Check sheet for the drawn part. Datum: minimum x, y, z corner. Units: mm. A direction names the side the tool comes from. Round coordinates to 2 decimals unless told otherwise and drop trailing zeros. Write each loop counter-clockwise with the first axis right and the second up, starting at its lowest first coordinate (ties: lowest second). Pieces come first, ordered by that corner, then holes. Notation, with made-up numbers: (56.25, 8) -> (65.25, 8) arc R15 cw to (65.25, 29) -> close; hole circle Ø5 at (79, -36). An arc over 180 degrees is marked (long way). Use a Markdown table: item, result.
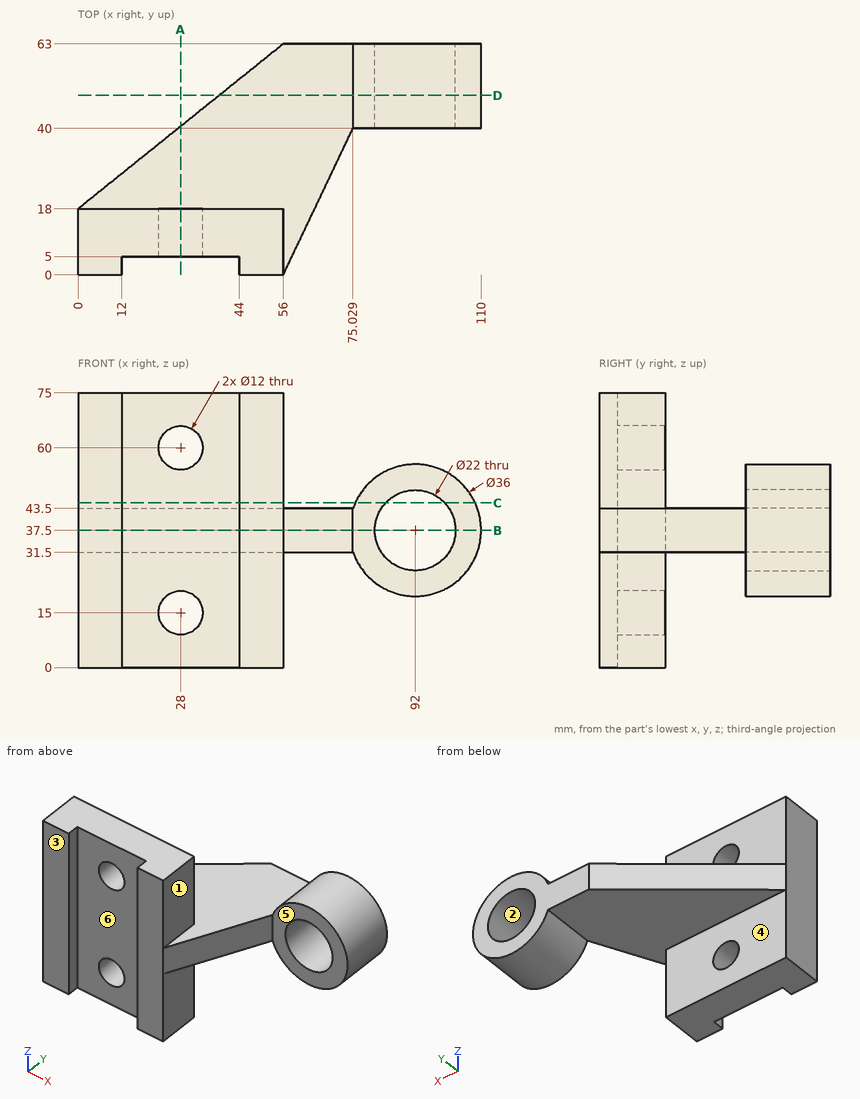
(1) Release check for a two-part mould opening along X. For the marked faces 1, 2 and 3 record: +X half, -X half, draft (parallel to the pull), parting line (faces both ways), or undercut.
A:
| item | result |
|---|---|
| face 1 | +X half |
| face 2 | undercut |
| face 3 | draft |
(2) Gauge pin test, flat ends, axial feed: pin 1 Ø1 at (x, y) = (58.5, 19) entering from -Z; pin 2 Ø17.5 at (x, z) = (89, 34) entering from -Y; pin 3 Ø4 at (y, z) = (3, 38.5) entering from +X. Record the tip position at first contact, or that the pin passes through.
A:
| item | result |
|---|---|
| pin 1 | stops at z = 31.5 |
| pin 2 | stops at y = 40 |
| pin 3 | stops at x = 58.38 |
(3) Thickness scan on line 1 (X direction, y = 10, z = 15); line 2 (Y direction, x = 39.5, z = 4.5); line 3 (Z direction, x = 73.5, y = 37). Record the ranges inside material, lowest first.
A:
| item | result |
|---|---|
| line 1 | x = 0 to 22, 34 to 56 |
| line 2 | y = 5 to 18 |
| line 3 | z = 31.5 to 43.5 |
(4) Section check A-A on x = 28. Record the cut outline in (y, z).
A:
| item | result |
|---|---|
| outline | (5, 0) -> (18, 0) -> (18, 9) -> (5, 9) -> close; (5, 21) -> (18, 21) -> (18, 31.5) -> (40.5, 31.5) -> (40.5, 43.5) -> (18, 43.5) -> (18, 54) -> (5, 54) -> close; (5, 66) -> (18, 66) -> (18, 75) -> (5, 75) -> close |
(5) Section check D-D on y = 49. Record the cut outline in (x, z), plus the area to 3 significant figures.
A:
| item | result |
|---|---|
| outline | (38.58, 31.5) -> (75.03, 31.5) arc R18 ccw (long way) to (75.03, 43.5) -> (38.58, 43.5) -> close; hole circle Ø22 at (92, 37.5) |
| area | 1,070 mm2 |
(6) Section check C-C on z = 45. Record the cut outline in (x, y), plus the area to 3 significant figures.
A:
| item | result |
|---|---|
| outline | (0, 0) -> (12, 0) -> (12, 5) -> (44, 5) -> (44, 0) -> (56, 0) -> (56, 18) -> (0, 18) -> close; (75.64, 40) -> (83.95, 40) -> (83.95, 63) -> (75.64, 63) -> close; (100.05, 40) -> (108.36, 40) -> (108.36, 63) -> (100.05, 63) -> close |
| area | 1,230 mm2 |
(7) Access from +Z, -Z, +X, -X, +Y, -Y to the whole of each face (thin tool, end or side, straight path). Record for the marked faces 4, 5 and 6.
A:
| item | result |
|---|---|
| face 4 | -Z, +X, -X, +Y |
| face 5 | +Z, -Z, +X, -Y |
| face 6 | +Z, -Z, -Y |
(8) Section check B-B on z = 37.5. Record the cut outline in (x, y).
A:
| item | result |
|---|---|
| outline | (0, 0) -> (12, 0) -> (12, 5) -> (44, 5) -> (44, 0) -> (56, 0) -> (75.03, 40) -> (81, 40) -> (81, 63) -> (56, 63) -> (0, 18) -> close; (103, 40) -> (110, 40) -> (110, 63) -> (103, 63) -> close |
